from build123d import *

# Parameters (mm, degrees)
F1_DEPTH = 10


with BuildPart() as f1:
    # F0 (on Top) → F1 (new body)
    with BuildSketch(Plane.XY):
        with BuildLine():
            ThreePointArc((300, 250), (285.355339, 285.355339), (250, 300))
            Line((250, 300), (-250, 300))
            ThreePointArc((-250, 300), (-285.355339, 285.355339), (-300, 250))
            Line((-300, 250), (-300, 150))
            Line((-300, 150), (-210.945189, 150))
            Line((-210.945189, 150), (-210.945189, -150))
            Line((-210.945189, -150), (-300, -150))
            Line((-300, -150), (-300, -250))
            ThreePointArc((-300, -250), (-285.355339, -285.355339), (-250, -300))
            Line((-250, -300), (250, -300))
            ThreePointArc((250, -300), (285.355339, -285.355339), (300, -250))
            Line((300, -250), (300, -150))
            Line((300, -150), (210.945189, -150))
            Line((210.945189, -150), (210.945189, 150))
            Line((210.945189, 150), (300, 150))
            Line((300, 150), (300, 250))
        make_face()
    extrude(amount=F1_DEPTH)


solid = f1.part
Input: part model. Units: mm. Frame: model coordinates. Coordinates: 2 decimals unless noted, no trailing zeros. Loops run counter-clockwise (first coordinate to the right, second up) from the corner with the lowest first, then second, coordinate; pieces in that order, holes last.
(1) Section A-A on x = 227. Return the cut outline in (y, z).
(2) Material intervals for probe 1 along X at (y, z) = (54.5, 7); probe 2 along Y at (x, z) = (-253.5, 7.25); probe 3 along Y at (x, z) = (-256, 7), sorted ascending.
(3) First-contact query: pin 1 Ø5 at (x, z) = (-270.5, 5) entering from -Y; pin 2 Ø3 at (x, z) = (-274, 6) entering from +Y; pin 3 Ø3 at (y, z) = (55.5, 5) entering from +X. Flat tips, straight axial feed; report the tip coordinate or a pass-through.
(4) Section C-C on y = -97. Return the cut outline in (x, z), then the cut area to 3 significant figures.
(5) Section B-B on z = 4.75. Return the cut outline in (x, y).
Data:
1. outline: (-300, 0) - (-150, 0) - (-150, 10) - (-300, 10) - close; (150, 0) - (300, 0) - (300, 10) - (150, 10) - close
2. probe 1: x = -210.95 to 210.95
2. probe 2: y = -299.88 to -150, 150 to 299.88
2. probe 3: y = -299.64 to -150, 150 to 299.64
3. pin 1: stops at y = -296.65
3. pin 2: stops at y = 294.65
3. pin 3: stops at x = 210.95
4. outline: (-210.95, 0) - (210.95, 0) - (210.95, 10) - (-210.95, 10) - close
4. area: 4,220 mm2
5. outline: (-300, -250) arc R50 ccw to (-250, -300) - (250, -300) arc R50 ccw to (300, -250) - (300, -150) - (210.95, -150) - (210.95, 150) - (300, 150) - (300, 250) arc R50 ccw to (250, 300) - (-250, 300) arc R50 ccw to (-300, 250) - (-300, 150) - (-210.95, 150) - (-210.95, -150) - (-300, -150) - close
